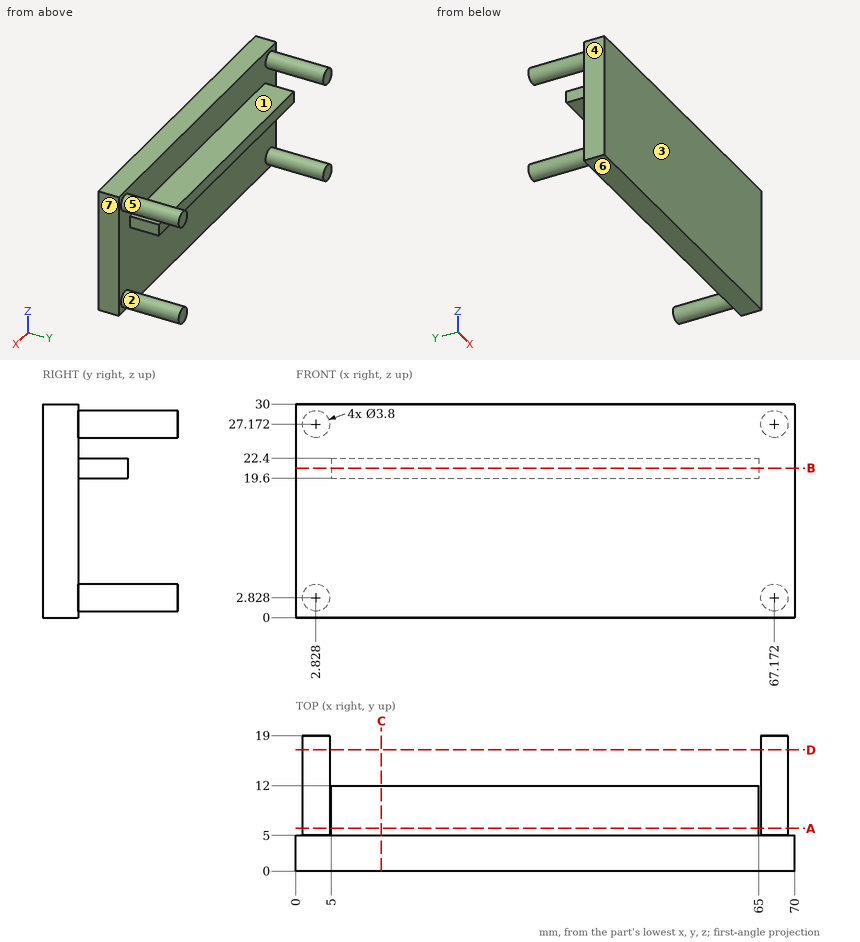
Print and shaded views of the part. All mm, measured from the part's lowest x, y and z. A direction names the side the tool comes from. Round coordinates to 2 decimals unless told otherwise and drop trailing zeros. Write each loop counter-clockwise with the first axis right and the second up, starting at its lowest first coordinate (ties: lowest second). Pieces come first, ordered by that corner, then holes. Notation, with made-up numbers: (19.25, -21.75) -> (69.25, -21.75) arc R9 cw to (69.25, -10.75) -> close; hole circle Ø10 at (76, -38.5). An arc over 180 degrees is marked (long way). Answer in a Markdown table with one row per item. Add a question column.
Item 1: Drill centre lines: line 1 (Y direction, x = 18, z = 23.5); line 2 (Y direction, x = 10, z = 21); line 3 (X direction, y = 8, z = 4.25) (1 decimal). Where is each one in solid material? Low to high. Write a range as from..to.
Item 2: Mould opens along X. For the marked faces 4, 5, 6 and 7 say: pulls with the +X half, pulls with the -X half, needs draft (parallel to the pull), parting line crosses it, or undercut.
Item 3: Saw through at A-A, the plane y = 6. Write the cut outline in (x, z).
Item 4: Saw through at C-C, the plane x = 12. Write the cut outline in (y, z).
Item 5: Drop flat-ended pins along their axis: pin 1 Ø1.5 at (x, z) = (52.5, 7.5) entering from -Y; pin 2 Ø3 at (x, z) = (34.5, 21) entering from +Y; pin 3 Ø1.4 at (y, z) = (8, 21) entering from +X; pin 4 Ø1.5 at (y, z) = (6.5, 13.5) entering from +X. Give the stop position or say it passes through.
Item 6: Saw through at D-D, the plane y = 17. Write the cut outline in (x, z).
Item 7: Saw through at B-B, the plane z = 21. Write the cut outline in (x, y).
Item 8: Which spindle directions (+Z, -Z, +X, -X, +Y, -Y) get a long thin tool onto all of the face, cutting with end or side? Do the marked faces 1, 2 and 3. Say none if no direction does.
Findings below:
| question | item | result |
|---|---|---|
| 1 | line 1 | y = 0..5 |
| 1 | line 2 | y = 0..12 |
| 1 | line 3 | x = 1.6..4.1, 65.9..68.4 |
| 2 | face 4 | pulls with the -X half |
| 2 | face 5 | undercut |
| 2 | face 6 | needs draft |
| 2 | face 7 | pulls with the +X half |
| 3 | outline | circle Ø3.8 at (2.83, 2.83); circle Ø3.8 at (2.83, 27.17); (5, 19.6) -> (65, 19.6) -> (65, 22.4) -> (5, 22.4) -> close; circle Ø3.8 at (67.17, 2.83); circle Ø3.8 at (67.17, 27.17) |
| 4 | outline | (0, 0) -> (5, 0) -> (5, 19.6) -> (12, 19.6) -> (12, 22.4) -> (5, 22.4) -> (5, 30) -> (0, 30) -> close |
| 5 | pin 1 | stops at y = 0 |
| 5 | pin 2 | stops at y = 12 |
| 5 | pin 3 | stops at x = 65 |
| 5 | pin 4 | passes through |
| 6 | outline | circle Ø3.8 at (2.83, 2.83); circle Ø3.8 at (2.83, 27.17); circle Ø3.8 at (67.17, 2.83); circle Ø3.8 at (67.17, 27.17) |
| 7 | outline | (0, 0) -> (70, 0) -> (70, 5) -> (65, 5) -> (65, 12) -> (5, 12) -> (5, 5) -> (0, 5) -> close |
| 8 | face 1 | +Z, +X, -X, +Y |
| 8 | face 2 | +Y |
| 8 | face 3 | +Z, -Z, +X, -X, -Y |
